Could you check a few things on this model? Use its own coordinates, in mm. Face numbers are marked on the shaded views. A direction names the side the tool comes from. Give positions to 0.01 mm unless a question says otherwise; leave off trailing zeros. Write each loop counter-clockwise with the first axis right and the second up, starting at its lowest first coordinate (ties: lowest second). Pieces come first, ordered by that corner, then holes. Notation, with made-up numbers: M 88,59.25 L 108,59.25 A7 cw 108,71.25 Z; hole C 80.25,28 d2. An arc over 180 degrees is marked long. One line per item, written item: value.
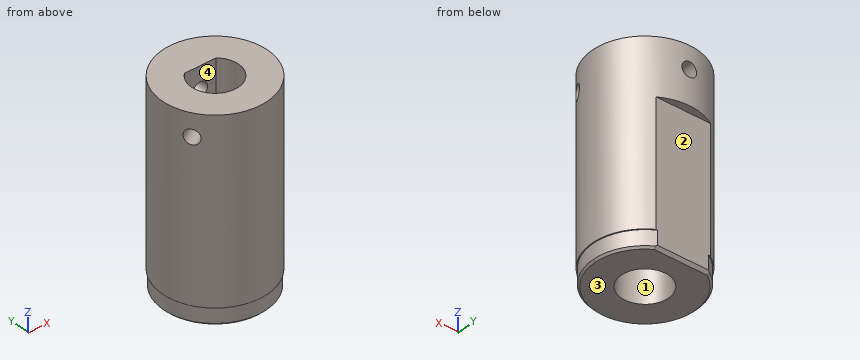
```python
from build123d import *

# Parameters (mm, degrees)
SKETCH_2_R               = 9.36
SKETCH_2_R_2             = 4.2
EXTRUDE_1_DEPTH          = 35
EXTRUDE_START            = -10
EXTRUDE_2_DEPTH          = 10
CUT_EXTRUDE_1_REACH      = 42.78
SKETCH_3_R               = 1.3
PATTERN_CIRCULAR_1_COUNT = 3
CUT_EXTRUDE_2_DEPTH      = 25
CHAMFER_1_SIZE           = 0.5
SKETCH_7_R               = 9.5
SKETCH_7_R_2             = 9.2
CUT_EXTRUDE_3_DEPTH      = 3


with BuildPart() as part:
    # Эскиз2 → Бобышка-Вытянуть1 (new body)
    with BuildSketch(Plane.XY):
        Circle(SKETCH_2_R)
        Circle(SKETCH_2_R_2, mode=Mode.SUBTRACT)
    extrude(amount=EXTRUDE_1_DEPTH)

    # Эскиз4 → Бобышка-Вытянуть2 (add)
    with BuildSketch(Plane.XY.offset(35).offset(EXTRUDE_START)):
        with BuildLine():
            Line((-2.833725463, 3.1), (2.833725463, 3.1))
            ThreePointArc((2.833725463, 3.1), (0, 4.2), (-2.833725463, 3.1))
        make_face()
    extrude(amount=EXTRUDE_2_DEPTH)

    # Эскиз3 → Вырез-Вытянуть1 (cut, up to next)
    with BuildSketch(Plane(origin=(0, 9.36, 0), x_dir=(1, 0, 0), z_dir=(0, 1, 0)), mode=Mode.PRIVATE) as cut_extrude_1_sk1:
        with Locations(Location((0, -31, 0), (0, 0, 270))):
            Circle(SKETCH_3_R)
    cut_extrude_1_tool1 = extrude(cut_extrude_1_sk1.sketch, amount=-CUT_EXTRUDE_1_REACH, mode=Mode.PRIVATE) & part.part
    cut_extrude_1 = cut_extrude_1_tool1.solids().sort_by_distance((0, 9.36, 31))[0]
    add(cut_extrude_1, mode=Mode.SUBTRACT)

    # Круговой массив1: Вырез-Вытянуть1 ×3 about axis
    pattern_circular_1_axis = Axis((0, 0, 35), (0, 0, -1))
    for i in range(1, PATTERN_CIRCULAR_1_COUNT):
        add(cut_extrude_1.rotate(pattern_circular_1_axis, i * 360 / PATTERN_CIRCULAR_1_COUNT), mode=Mode.SUBTRACT)

    # Эскиз5 → Вырез-Вытянуть2 (cut)
    with BuildSketch(Plane(origin=(0, 0, 0), x_dir=(-1, 0, 0), z_dir=(0, 0, -1))):
        with BuildLine():
            Line((-4.858971084, 8), (4.858971084, 8))
            ThreePointArc((4.858971084, 8), (0, 9.36), (-4.858971084, 8))
        make_face()
    extrude(amount=-CUT_EXTRUDE_2_DEPTH, mode=Mode.SUBTRACT)

    # Фаска1
    chamfer_1_edges = [part.edges().sort_by_distance(p)[0] for p in [
        (-4.589642178, -8.157498678, 0),
        (0, 8, 0),
    ]]
    chamfer(chamfer_1_edges, length=CHAMFER_1_SIZE)

    # Эскиз7 → Вырез-Вытянуть3 (cut)
    with BuildSketch(Plane(origin=(0, 0, 0), x_dir=(-1, 0, 0), z_dir=(0, 0, -1))):
        Circle(SKETCH_7_R)
        Circle(SKETCH_7_R_2, mode=Mode.SUBTRACT)
    extrude(amount=-CUT_EXTRUDE_3_DEPTH, mode=Mode.SUBTRACT)


solid = part.part
```
1) If we section it at C-C, the plane z = 31: Write out the boundary of the cut face in (x, y).
Outcome:
outline: M -8.68,-3.51 L -4.11,-0.87 A4.2 cw -2.83,3.1 L -1.3,3.1 L -1.3,9.27 A9.36 ccw Z; M -7.38,-5.76 A9.36 ccw 7.38,-5.76 L 2.81,-3.12 A4.2 cw -2.81,-3.12 Z; M 1.3,3.1 L 2.83,3.1 A4.2 cw 4.11,-0.87 L 8.68,-3.51 A9.36 ccw 1.3,9.27 Z
2) On a 3-axis mill with a long thin cutter (end or side, diameter ignored), from which of +Z, -Z, +X, -X, +Y, -Y can I reach the whole of each face in a straight line? I mean the marked faces 1, 2, 3 and 4. Say none if no direction works.
Outcome:
face 1: -Z
face 2: -Z, +X, -X, +Y
face 3: -Z, +X, -X, +Y, -Y
face 4: +Z, -Z
3) If we section it at D-D, the plane z = 5: Write out the boundary of the cut face in (x, y).
Outcome:
outline: M -4.86,8 A9.36 ccw long 4.86,8 Z; hole C 0,0 d8.4
4) Please list where these lines run through material, in increasing order: L1, parallel to Z at x = 0, y = 7; L2, parallel to X at y = 0, z = 10.5; L3, parallel to Y at x = 0, z = 14. Write a range as from..to.
Outcome:
L1: z = 0..29.7, 32.3..35
L2: x = -9.36..-4.2, 4.2..9.36
L3: y = -9.36..-4.2, 4.2..8
5) If we section it at A-A, the plane x = 0: Write out the boundary of the cut face in (y, z), then the cut area to 3 significant figures.
Outcome:
outline: M -9.36,3 L -9.2,3 L -9.2,0.34 L -8.86,0 L -4.2,0 L -4.2,35 L -9.36,35 Z; M 3.1,25 L 4.2,25 L 4.2,0 L 7.5,0 L 8,0.5 L 8,25 L 9.36,25 L 9.36,29.7 L 3.1,29.7 Z; M 3.1,32.3 L 9.36,32.3 L 9.36,35 L 3.1,35 Z
area: 321 mm^2
6) If we section it at B-B, the plane z = 25.5: Write out the boundary of the cut face in (x, y), then the cut area to 3 significant figures.
Outcome:
outline: C 0,0 d18.72; hole M -2.83,3.1 A4.2 ccw long 2.83,3.1 Z
area: 224 mm^2
7) I'm going to push flat-ended pins straight in: pin 1 (6.5 mm diameter, centred on x = 0, y = 0, fed in from -Z); pin 2 (2 mm diameter, centred on y = 1.5, z = 18, fed in from +X); pin 3 (3 mm diameter, centred on y = -4, z = 15.5, fed in from +X). Where does each tip first touch, or does it pass through?
Outcome:
pin 1: stops at z = 25
pin 2: stops at x = 9.35
pin 3: stops at x = 9.02
